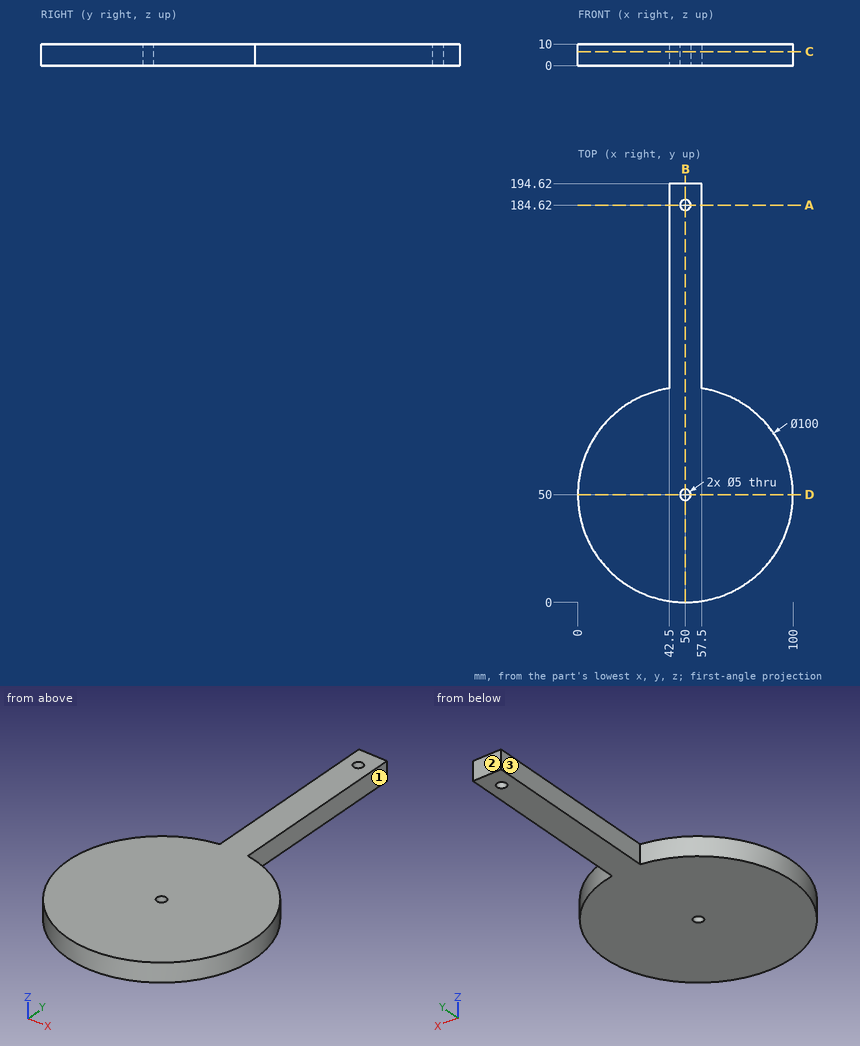
Design review of the part shown in the three views and the two pictorial views. Dimensions are in mm from the part's minimum x, y and z. A direction names the side the tool comes from. Give positions to 0.01 mm unless a question says otherwise; leave off trailing zeros. Loops run counter-clockwise (first coordinate to the right, second up) from the corner with the lowest first, then second, coordinate; pieces in that order, holes last. Notation, with made-up numbers: M 48,57.25 L 107,57.25 A23 cw 107,81.25 Z; hole C -19.5,-36.75 d11. An arc over 180 degrees is marked long. Put each result on its own line as item: value. Start each with the question number.
(1) Machinability: for the marked faces 1, 2 and 3, which of the approach directions +Z, -Z, +X, -X, +Y, -Y give a long, thin tool a straight path to every point of the face, cutting with its end or side? Answer none if there is none.
(2) For pin 1 (5 mm diameter, centred on x = 31, z = 5, fed in from -Y); pin 2 (6 mm diameter, centred on x = 20.5, z = 6.5, fed in from +Y); pin 3 (1.5 mm diameter, centred on x = 66, z = 2, fed in from -Y); pin 4 (1 mm diameter, centred on x = 48.5, y = 94.5, fed in from -Z), all flat-tipped, find the tip position at first contact; note any pin that passes through.
(3) Add section A-A, the plane y = 184.62. Write out the cut boundary in (x, z).
(4) Wall thickness on L1, parallel to Y at x = 50, z = 6.25; L2, parallel to X at y = 184.62, z = 6.25; L3, parallel to X at y = 101.5, z = 2.5: over which ranges is each line inside the solid? List them lowest first.
(5) Add section C-C, the plane z = 6.5. Write out the cut boundary in (x, y), then the cut area to 3 significant figures.
(6) Add section B-B, the plane x = 50. Write out the cut boundary in (y, z).
(7) Add section D-D, the plane y = 50. Write out the cut boundary in (x, z).
Result:
1. face 1: +Z, -Z, +X, +Y
1. face 2: +Z, -Z, +X, -X, +Y
1. face 3: +Z, -Z, -X, +Y
2. pin 1: stops at y = 2.8
2. pin 2: stops at y = 92.4
2. pin 3: stops at y = 2.38
2. pin 4: stops at z = 0
3. outline: M 42.5,0 L 47.5,0 L 47.5,10 L 42.5,10 Z; M 52.5,0 L 57.5,0 L 57.5,10 L 52.5,10 Z
4. L1: y = 0 to 47.5, 52.5 to 182.12, 187.12 to 194.62
4. L2: x = 42.5 to 47.5, 52.5 to 57.5
4. L3: x = 42.5 to 57.5
5. outline: M 42.5,99.43 A50 ccw long 57.5,99.43 L 57.5,194.62 L 42.5,194.62 Z; hole C 50,50 d5; hole C 50,184.62 d5
5. area: 9,240 mm^2
6. outline: M 0,0 L 47.5,0 L 47.5,10 L 0,10 Z; M 52.5,0 L 182.12,0 L 182.12,10 L 52.5,10 Z; M 187.12,0 L 194.62,0 L 194.62,10 L 187.12,10 Z
7. outline: M 0,0 L 47.5,0 L 47.5,10 L 0,10 Z; M 52.5,0 L 100,0 L 100,10 L 52.5,10 Z
